Verification items for this drawing (mm, ordinates from the low corner). Coordinates: 2 decimals unless noted, no trailing zeros. Order: outer loops, then holes, each group sorted by start corner. A loop starts at its lowest first (then second) coordinate and runs counter-clockwise, first axis right, second up. Notation, with made-up numbers: M 4,14 L 53,14 A30 cw 53,38 Z; hole C 75,9 d6. An arc over 180 degrees is marked long. Return JSON: item names as keys, results as strings. Group by question number.
1. Gauge pin test, flat end, axial feed: pin 1 (4 mm diameter, centred on x = 158.5, z = 121, fed in from -Y). Record the tip position at first contact, or that the pin passes through.
2. Section check A-A, the plane y = 3. Record the cut outline in (x, z), plus the area to 3 significant figures.
3. Section check D-D, the plane x = 151. Record the cut outline in (y, z).
4. Section check C-C, the plane z = 38.1. Record the cut outline in (x, y), plus the area to 3 significant figures.
5. Material ranges on line 1 along Z through (x, y) = (38.1, 5); line 2 along Z through (x, y) = (100, 0.75); line 3 along Z through (x, y) = (38.1, 7), recorded low to high.
6. Section check B-B, the plane x = 38.1. Record the cut outline in (y, z), plus the area to 3 significant figures.
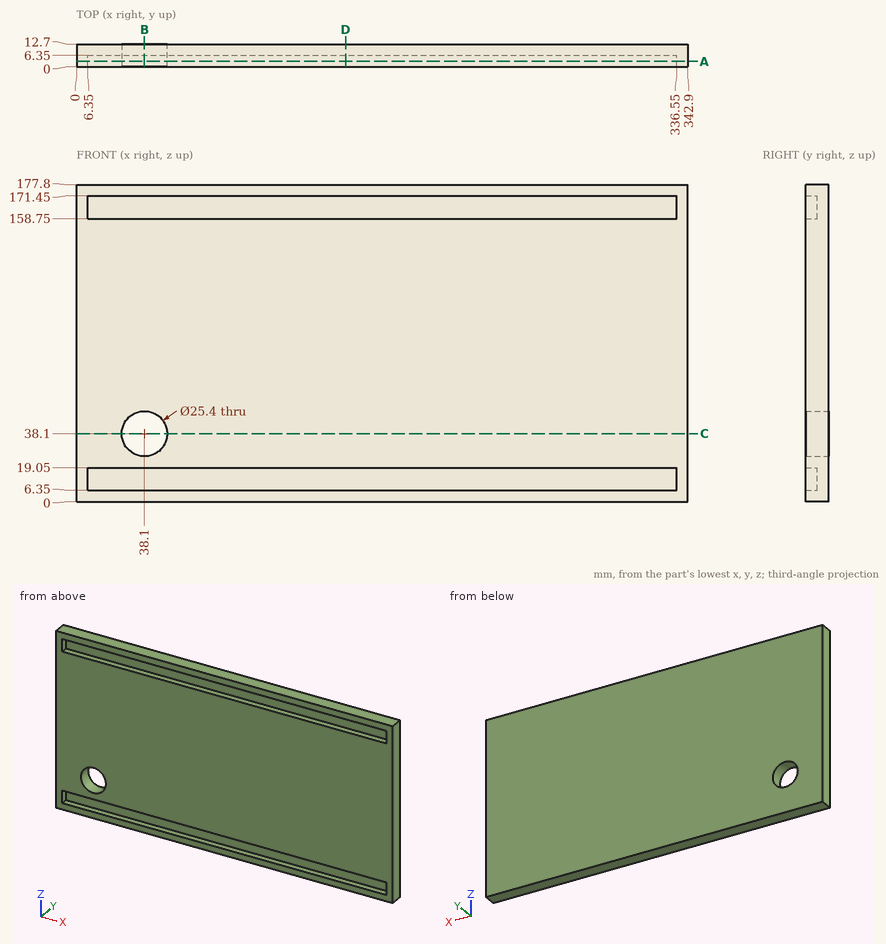
Answers follow:
{
 "1": {"pin 1": "y = 0"},
 "2": {"outline": "M 0,0 L 342.9,0 L 342.9,177.8 L 0,177.8 Z; hole M 6.35,6.35 L 336.55,6.35 L 336.55,19.05 L 6.35,19.05 Z; hole M 6.35,158.75 L 336.55,158.75 L 336.55,171.45 L 6.35,171.45 Z; hole C 38.1,38.1 d25.4", "area": "52,100 mm^2"},
 "3": {"outline": "M 0,0 L 12.7,0 L 12.7,177.8 L 0,177.8 L 0,171.45 L 6.35,171.45 L 6.35,158.75 L 0,158.75 L 0,19.05 L 6.35,19.05 L 6.35,6.35 L 0,6.35 Z"},
 "4": {"outline": "M 0,0 L 25.4,0 L 25.4,12.7 L 0,12.7 Z; M 50.8,0 L 342.9,0 L 342.9,12.7 L 50.8,12.7 Z", "area": "4,030 mm^2"},
 "5": {"line 1": "0 to 6.35, 19.05 to 25.4, 50.8 to 158.75, 171.45 to 177.8", "line 2": "0 to 6.35, 19.05 to 158.75, 171.45 to 177.8", "line 3": "0 to 25.4, 50.8 to 177.8"},
 "6": {"outline": "M 0,0 L 12.7,0 L 12.7,25.4 L 0,25.4 L 0,19.05 L 6.35,19.05 L 6.35,6.35 L 0,6.35 Z; M 0,50.8 L 12.7,50.8 L 12.7,177.8 L 0,177.8 L 0,171.45 L 6.35,171.45 L 6.35,158.75 L 0,158.75 Z", "area": "1,770 mm^2"}
}
